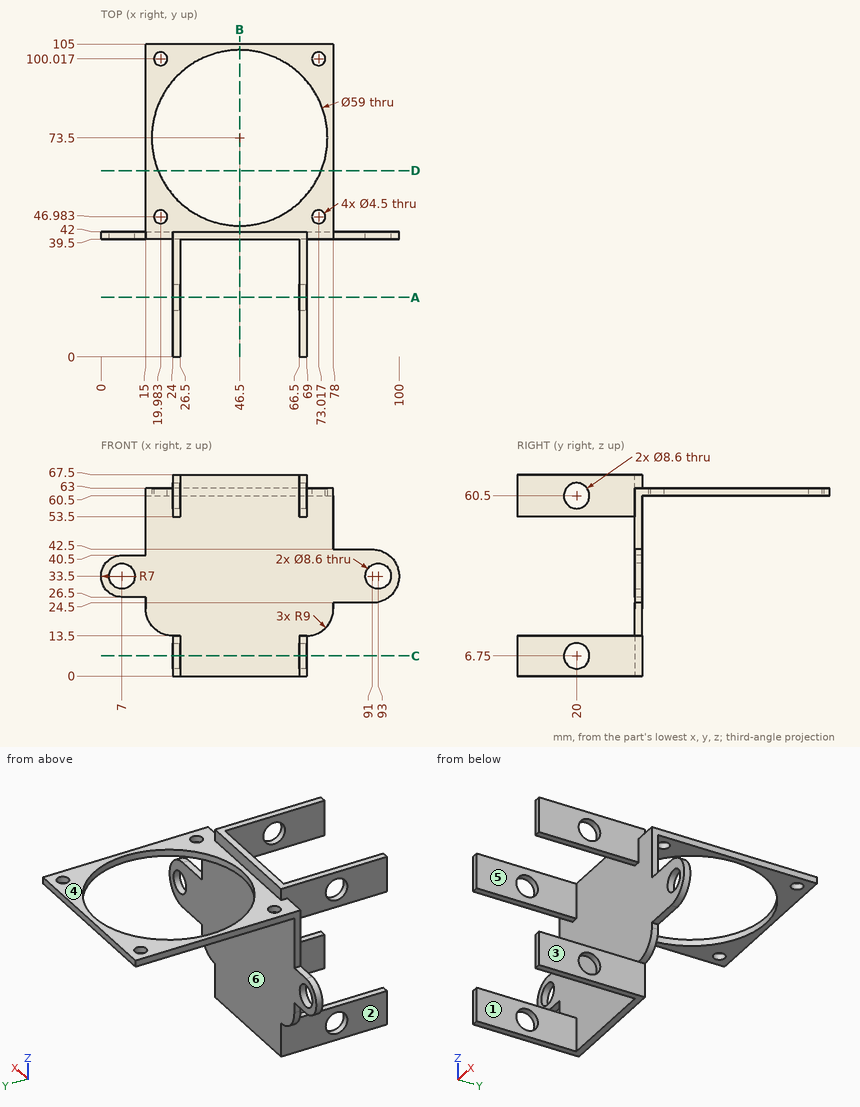
Geometry check sheet. Reference: drawing and pictorial views, mm from the part's lowest x, y, z. A direction names the side the tool comes from. Round coordinates to 2 decimals unless told otherwise and drop trailing zeros. Order: outer loops, then holes, each group sorted by start corner. A loop starts at its lowest first (then second) coordinate and runs counter-clockwise, first axis right, second up.
Q1. Cross-section at B-B, the plane x = 46.5. Enter the section's corners in (y, z), plus the area to 3 significant figures.
Filled sheet:
outline: (39.5, 0) - (42, 0) - (42, 60.5) - (44, 60.5) - (44, 63) - (42, 63) - (42, 67.5) - (39.5, 67.5) - close; (103, 60.5) - (105, 60.5) - (105, 63) - (103, 63) - close
area: 179 mm2
Q2. Cross-section at C-C, the plane z = 6.75. Enter the section's corners in (x, y), plus the area to 3 significant figures.
Filled sheet:
outline: (24, 0) - (26.5, 0) - (26.5, 15.7) - (24, 15.7) - close; (24, 24.3) - (26.5, 24.3) - (26.5, 39.5) - (66.5, 39.5) - (66.5, 24.3) - (69, 24.3) - (69, 42) - (24, 42) - close; (66.5, 0) - (69, 0) - (69, 15.7) - (66.5, 15.7) - close
area: 267 mm2
Q3. Cross-section at D-D, the plane y = 62.5. Enter the section's corners in (x, z).
Filled sheet:
outline: (15, 60.5) - (19.13, 60.5) - (19.13, 63) - (15, 63) - close; (73.87, 60.5) - (78, 60.5) - (78, 63) - (73.87, 63) - close
Q4. Scan lines: L1, parallel to X at y = 38.5, z = 6.5; L2, parallel to Y at x = 72, z = 39.5; L3, parallel to Y at x = 46.5, z = 62.15. Record each from-to range of solid material in increasing order.
Filled sheet:
L1: x = 24 to 26.5, 66.5 to 69
L2: y = 39.5 to 42
L3: y = 39.5 to 44, 103 to 105
Q5. Draft check along X on the marked faces 1, 2, 3 and 4. Enter one of: pulls with the +X half, pulls with the -X half, needs draft (parallel to the pull), parting line crosses it, or undercut.
Filled sheet:
face 1: undercut
face 2: pulls with the -X half
face 3: pulls with the +X half
face 4: needs draft
Q6. Cross-section at A-A, the plane y = 20. Give the number of separate pieces and of enclosed holes in the cut face.
Filled sheet:
separate pieces: 8
enclosed holes: 0
Q7. Depth check by flat-ended pin: P1, Ø5, axis at x = 19.98, y = 100.02, coming from the -Z side; P2, Ø20, axis at x = 42.5, z = 45.5, coming from the -Y side; P3, Ø4, axis at x = 73.02, y = 100.02, coming from the +Z side; P4, Ø11, axis at y = 12, z = 6.5, coming from the -X side. Enter the tip coordinate at first touch or a pass-through.
Filled sheet:
P1: stops at z = 60.5
P2: stops at y = 39.5
P3: passes through
P4: stops at x = 24
Q8. Set-up check for the marked faces 5 and 6: record each of +Z, -Z, +X, -X, +Y, -Y from which the full face is reachable in a straight line by a thin tool's end or side.
Filled sheet:
face 5: +Z, -Z, -Y
face 6: -Z, +X, -X, +Y
